from build123d import *

# Parameters (mm, degrees)
F0_W     = 38.1
F0_H     = 38.1
F1_DEPTH = 38.1
F5_DEPTH = 38.1
F7_DEPTH = 38.1
F8_W     = 25.4
F8_H     = 7.62
F9_DEPTH = 38.1


with BuildPart() as f1:
    # F0 (on Front) → F1 (new body)
    with BuildSketch(Plane.XZ):
        with Locations((19.05, 19.05)):
            Rectangle(F0_W, F0_H)
    extrude(amount=F1_DEPTH)

    # F4 (on offset) → F5 (cut)
    with BuildSketch(Plane.YZ.offset(38.1)):
        Polygon((-6.35, 0), (0, 0), (0, 38.1), align=None)
        Polygon((-11.43, 17.476514), (-6.35, 38.1), (-31.75, 38.1), (-26.67, 15.875), (-21.59, 28.575), (-16.51, 28.575), align=None)
        Polygon((-31.75, 0), (-38.1, 38.1), (-38.1, 0), align=None)
        Polygon((-25.4, 0), (-12.7, 0), (-19.05, 15.875), align=None)
    extrude(amount=-F5_DEPTH, mode=Mode.SUBTRACT)

    # F6 (on Front) → F7 (cut)
    with BuildSketch(Plane.XZ):
        Polygon((11.43, 22.225), (6.35, 0), (31.75, 0), (26.67, 22.225), (21.59, 9.525), (16.51, 9.525), align=None)
        Polygon((31.75, 38.1), (38.1, 0), (38.1, 38.1), align=None)
        Polygon((25.4, 38.1), (12.7, 38.1), (19.05, 25.139847), align=None)
        Polygon((6.35, 38.1), (0, 38.1), (0, 0), align=None)
    extrude(amount=F7_DEPTH, mode=Mode.SUBTRACT)

    # F8 (on offset) → F9 (cut)
    with BuildSketch(Plane.XY.offset(38.1)):
        with Locations((25.4, -11.43)):
            Rectangle(F8_W, F8_H)
        with Locations((12.7, -26.67)):
            Rectangle(F8_W, F8_H)
    extrude(amount=-F9_DEPTH, mode=Mode.SUBTRACT)


solid = f1.part
Read the model definition and answer for the solid it produces. Units are mm, in the model's axes. A direction names the side the tool comes from. Round coordinates to 2 decimals unless told otherwise and drop trailing zeros. Write each loop counter-clockwise with the first axis right and the second up, starting at its lowest first coordinate (ties: lowest second). Pieces come first, ordered by that corner, then holes.
Q1. Find section D-D on z = 8. Determine the outline of the cut face in (x, y).
Values:
outline: (1.33, -33.08) - (8.18, -33.08) - (8.18, -30.48) - (1.33, -30.48) - close; (1.33, -22.86) - (8.18, -22.86) - (8.18, -22.2) - (1.33, -22.2) - close; (1.33, -15.9) - (8.18, -15.9) - (8.18, -5.02) - (1.33, -5.02) - close; (29.92, -33.08) - (36.77, -33.08) - (36.77, -22.2) - (29.92, -22.2) - close; (29.92, -15.9) - (36.77, -15.9) - (36.77, -15.24) - (29.92, -15.24) - close; (29.92, -7.62) - (36.77, -7.62) - (36.77, -5.02) - (29.92, -5.02) - close
Q2. Straight lines are drawn through the part: line 1 (X direction, y = -17, z = 15); line 2 (Y direction, x = 3.5, z = 10.5); line 3 (Y direction, x = 10, z = 21). For each, find the intervals that lie inside material, in ascending order.
Values:
line 1: x = 2.5 to 9.78, 14.32 to 23.78, 28.32 to 35.6
line 2: y = -33.5 to -30.48, -22.86 to -21.2, -16.9 to -4.6
line 3: y = -35.25 to -30.48, -22.86 to -13.04, -10.56 to -2.85
Q3. Find section C-C on y = -4. Determine the outline of the cut face in (x, z) (3 decimals).
Values:
outline: (2.35, 14.1) - (9.573, 14.1) - (11.43, 22.225) - (14.68, 14.1) - (23.42, 14.1) - (26.67, 22.225) - (28.527, 14.1) - (35.75, 14.1) - (31.75, 38.1) - (25.4, 38.1) - (19.05, 25.14) - (12.7, 38.1) - (6.35, 38.1) - close
Q4. Flat-ended cylindrical pins translate along their axes: P1, Ø5.5, axis at x = 9, z = 12.5, coming from the -Y side; P2, Ø1.5, axis at y = -11, z = 21, coming from the -X side; P3, Ø1, axis at x = 18.5, y = -16, coming from the -Z side (3 decimals); P4, Ø12, axis at x = 7, y = -32.5, coming from the -Z side. Find the tip coordinate at first contact, or state that the pin passes through.
Values:
P1: stops at y = -34.29
P2: stops at x = 3.38
P3: stops at z = 9.525
P4: stops at z = 0
Q5. The mould has two halves that part along X. Classify faces 5 (the face through (22.18, -34.24, 31.53)), 6 (the face through (19.88, -19, 26.83)), 7 (the face through (19.32, -3.13, 19.32)), 8 (the face through (12.7, -9, 23)): released by +X, released by -X, zero draft, split by the parting line, or undercut.
Values:
face 5: undercut
face 6: undercut
face 7: zero draft
face 8: released by +X
Q6. A tool of negligible diameter and unlimited length cuts with its end or side. For faces 1 (the face through (15.83, -34.24, 31.71)), 2 (the face through (19, -16, 9.525)), 3 (the face through (25, -7.62, 20)), 4 (the face through (26.688, -15.884, 27.207)), from which of +Z, -Z, +X, -X, +Y, -Y can it reach the whole face along a straight path? Write none if from no direction.
Values:
face 1: +Z, +Y, -Y
face 2: -Z, +Y, -Y
face 3: +Z, -Z, +X
face 4: +Z, +X, -X
Q7. Find section B-B on z = 23.5. Determine the outline of the cut face in (x, y).
Values:
outline: (3.92, -35.67) - (34.18, -35.67) - (34.18, -28.41) - (25.4, -28.41) - (25.4, -30.48) - (3.92, -30.48) - close; (3.92, -22.86) - (25.4, -22.86) - (25.4, -23.62) - (34.18, -23.62) - (34.18, -15.24) - (12.7, -15.24) - (12.7, -14.19) - (3.92, -14.19) - close; (3.92, -9.95) - (12.7, -9.95) - (12.7, -7.62) - (34.18, -7.62) - (34.18, -2.43) - (3.92, -2.43) - close
Q8. Find section A-A on z = 35. Determine the outline of the cut face in (x, y).
Values:
outline: (5.83, -37.58) - (14.22, -37.58) - (14.22, -31.04) - (5.83, -31.04) - close; (5.83, -7.11) - (14.22, -7.11) - (14.22, -0.52) - (5.83, -0.52) - close; (23.88, -37.58) - (32.27, -37.58) - (32.27, -31.04) - (23.88, -31.04) - close; (23.88, -7.11) - (32.27, -7.11) - (32.27, -0.52) - (23.88, -0.52) - close
